Read the model definition and answer for the solid it produces. Units are mm, in the model's axes. Face numbers are marked on the shaded views. A direction names the side the tool comes from. Give positions to 0.01 mm unless a question says otherwise; leave off trailing zeros. Write each loop counter-clockwise with the first axis right and the second up, starting at its lowest first coordinate (ties: lowest second). Pieces come first, ordered by that corner, then holes. Notation, with made-up numbers: (63.5, 75) -> (101.5, 75) arc R23 cw to (101.5, 83) -> close; hole circle Ø5 at (67, -27.75). An arc over 180 degrees is marked (long way). Use a Markdown table: item, result.
Autodesk Inventor part; units mm, degrees
ref_plane "YZ Plane" through (0, 0, 0) normal (1, 0, 0) x (0, 1, 0)
ref_plane "XY Plane" through (0, 0, 0) normal (0, 0, 1) x (1, 0, 0)
sketch "Sketch1" plane through (0, 0, 0) normal (0, 0, 1) x (1, 0, 0)
  line L0 (0, 0) -> (1000, 0)
  line L1 (1000, 0) -> (1000, 1250)
  line L2 (1000, 1250) -> (0, 1250)
  line L3 (0, 1250) -> (0, 0)
  dimension "d0" = 1000
  dimension "d1" = 1250
extrude "Extrusion1" add sketch "Sketch1" along normal blind 100
sketch "Sketch2" plane through (0, 0, 0) normal (0, 0, -1) x (-1, 0, 0)
  line L0 (-1000, 1250) -> (0, 1250)
  circle A0 centre (-500, 1250) radius 500
  point P0 (0, 0)
  dimension "d4" = 1000
extrude "Extrusion2" add sketch "Sketch2" against normal blind 100 contours A0 L0 picked at (-386.6625, 1415.594)
sketch "Sketch3" plane through (0, 0, 0) normal (0, -1, 0) x (1, 0, 0)
  line L0 (0, 100) -> (1000, 100)
  circle A0 centre (350, 100) radius 50
  circle A1 centre (650, 100) radius 50
  line L1 (0, 0) -> (0, 100)
  line L2 (1000, 0) -> (1000, 100)
  point P0 (1000, 50)
  dimension "d7" = 100
  dimension "d8" = 100
  dimension "d9" = 350
  dimension "d10" = 350
extrude "Extrusion3" add sketch "Sketch3" against normal blind 1250
sketch "Sketch4" plane through (1000, 0, 100) normal (1, 0, 0) x (0, 0, -1)
  line L0 (0, 1250) -> (0, 0)
  circle A0 centre (0, 450) radius 50
  circle A1 centre (0, 850) radius 50
  line L1 (100, 0) -> (0, 0)
  line L2 (100, 1250) -> (0, 1250)
  dimension "d13" = 100
  dimension "d14" = 100
  dimension "d15" = 450
  dimension "d16" = 400
  dimension "d17" = 400
extrude "Extrusion4" add sketch "Sketch4" against normal blind 1000
sketch "Sketch5" plane through (0, 0, 100) normal (0, 0, 1) x (1, 0, 0)
  line L0 (700, 1250) -> (600, 1250)
  line L1 (400, 1250) -> (300, 1250)
  arc A0 (600, 1250) -> (400, 1250) centre (500, 1250) ccw
  arc A1 (700, 1250) -> (300.0458, 1245.6914) centre (500.0458, 1245.7187) ccw
  point P0 (0, 0)
  point P1 (300.0917, 1250)
  dimension "d20" = 100
  dimension "d21" = 200
extrude "Extrusion5" add sketch "Sketch5" along normal blind 50
sketch "Sketch6" plane through (1000, 0, 100) normal (1, 0, 0) x (0, 0, -1)
  line L0 (0, 900) -> (0, 1250)
  circle A0 centre (0, 1200) radius 50
  line L1 (100, 1250) -> (0, 1250)
  point P0 (100, 0)
  dimension "d24" = 100
  dimension "d25" = 50
extrude "Extrusion6" add sketch "Sketch6" against normal up to surface
sketch "Sketch7" plane through (0, 0, 0) normal (-1, 0, 0) x (0, 0, 1)
  line L0 (100, 900) -> (100, 1250)
  circle A0 centre (100, 1200) radius 50
  line L1 (0, 1250) -> (100, 1250)
  point P0 (0, 0)
  dimension "d28" = 100
  dimension "d29" = 50
extrude "Extrusion7" add sketch "Sketch7" against normal up to surface
ref_plane "Work Plane1" through (0, 1750, 0) normal (0, 1, 0) x (-1, 0, 0)
sketch "Sketch8" plane through (0, 1750, 0) normal (0, 1, 0) x (-1, 0, 0)
  line L0 (-400, 100) -> (-600, 100)
  circle A0 centre (-500, 100) radius 50
  point P0 (0, 0)
  dimension "d33" = 100
extrude "Extrusion8" add sketch "Sketch8" against normal up to surface
sketch "Sketch9" plane through (0, 0, 100) normal (0, 0, 1) x (1, 0, 0)
  line L0 (1000, 1150) -> (700, 1150)
  line L1 (900, 1150) -> (900, 902.0075)
  line L2 (1000, 900) -> (1000, 1150)
  line L3 (1000, 800) -> (700, 800)
  line L4 (900, 800) -> (900, 0)
  line L5 (0, 0) -> (1000, 0)
  line L6 (100, 0) -> (100, 1250)
  line L7 (0, 1250) -> (300, 1250)
  line L8 (0, 800) -> (0, 500)
  arc A0 (1000, 1250) -> (0, 1250) centre (500, 1250) ccw
  line L9 (0, 1250) -> (0, 0)
  line L10 (0, 1250) -> (0, 0)
  line L11 (700, 1250) -> (1000, 1250)
  line L12 (1000, 1250) -> (1000, 0)
  arc A1 (900, 1250) -> (100, 1250) centre (500, 1250) ccw
  point P0 (900, 1026.0038)
  point P1 (100, 625)
  dimension "d36" = 100
  dimension "d37" = 100
extrude "Extrusion9" add sketch "Sketch9" along normal blind 50 contours L11 A1 L7 A0
sketch "Sketch10" plane through (0, 0, 100) normal (0, 0, 1) x (1, 0, 0)
  arc A0 (900, 1250) -> (550, 1646.8627) centre (500, 1250) ccw
  line L0 (900, 1250) -> (900, 0)
  line L1 (1000, 0) -> (1000, 1250)
  line L2 (1000, 1250) -> (1000, 0)
  line L3 (1000, 1150) -> (700, 1150)
  line L4 (900, 1150) -> (1000, 1150)
  line L5 (0, 0) -> (1000, 0)
  line L6 (900, 0) -> (1000, 0)
extrude "Extrusion10" add sketch "Sketch10" along normal blind 50
sketch "Sketch11" plane through (0, 0, 100) normal (0, 0, 1) x (1, 0, 0)
  line L0 (100, 1250) -> (100, 0)
  line L1 (0, 0) -> (300, 0)
  line L2 (0, 0) -> (0, 1250)
  line L3 (0, 400) -> (0, 0)
  line L4 (0, 1250) -> (100, 1250)
  line L5 (0, 0) -> (100, 0)
extrude "Extrusion11" add sketch "Sketch11" along normal blind 50
sketch "Sketch12" plane through (0, 0, 100) normal (0, 0, 1) x (1, 0, 0)
  line L0 (700, 1250) -> (900, 1250)
  line L1 (900, 1250) -> (900, 1150)
  line L2 (900, 1150) -> (1000, 1150)
  line L3 (900, 1250) -> (1000, 1250)
  line L4 (1000, 1150) -> (1000, 1250)
  line L5 (1000, 1250) -> (900, 1250)
  point P0 (0, 0)
extrude "Extrusion12" add sketch "Sketch12" along normal blind 50
sketch "Sketch13" plane through (0, 0, 100) normal (0, 0, 1) x (1, 0, 0)
  line L0 (0, 1250) -> (0, 0)
  line L1 (0, 100) -> (1042, 100)
  line L2 (400, 0) -> (600, 0)
  line L3 (0, 0) -> (100, 0)
  line L4 (0, 100) -> (0, 0)
  line L5 (900, 0) -> (1000, 0)
  line L6 (0, 0) -> (1000, 0)
  line L7 (1000, 0) -> (1000, 100)
  line L8 (1000, 0) -> (1000, 1250)
  point P0 (500, 0)
  point P1 (521, 100)
  dimension "d46" = 100
extrude "Extrusion13" add sketch "Sketch13" along normal blind 50
sketch "Sketch14" plane through (0, 0, 0) normal (0, 0, -1) x (-1, 0, 0)
  arc A0 (-500, 1750) -> (-1000, 1250) centre (-500, 1250) ccw
  line L0 (-1000, 0) -> (-1000, 1250)
  line L1 (-1000, 1250) -> (-1000, 0)
  line L2 (0, 0) -> (-1000, 0)
  line L3 (-1000, 0) -> (0, 0)
  arc A1 (0, 1250) -> (-500, 1750) centre (-500, 1250) ccw
  line L4 (0, 0) -> (0, 1250)
  line L5 (0, 1250) -> (-1000, 1250)
  circle A2 centre (-500, 1250) radius 500
extrude "Extrusion14" add sketch "Sketch14" along normal blind 150
properties part number "WindowofShip11"
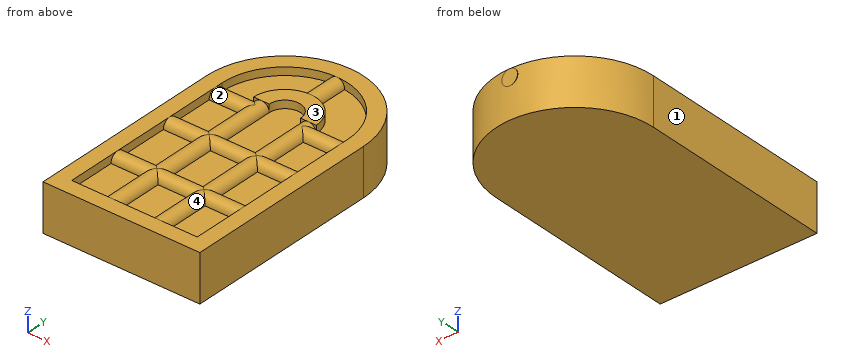
Item 1: For a pull along Y with two mould halves and no side action, classify the marked faces 3 and 4 as +Y half, -Y half, draft (parallel to the pull), parting line (faces both ways), or undercut.
Return value:
| item | result |
|---|---|
| face 3 | draft |
| face 4 | undercut |
Item 2: A tool of negligible diameter and unlimited length cuts with its end or side. For the marked faces 1 and 2, from which of +Z, -Z, +X, -X, +Y, -Y can it reach the whole face along a straight path? Write none if from no direction.
Return value:
| item | result |
|---|---|
| face 1 | +Z, -Z, -X, +Y, -Y |
| face 2 | +Z |
Item 3: A cutting plane is placed at B-B (z = -52). Give the vertices of the cut face in (x, y).
Return value:
| item | result |
|---|---|
| outline | (0, 0) -> (1000, 0) -> (1000, 1250) arc R500 ccw to (0, 1250) -> close |
Item 4: A cutting plane is placed at D-D (x = 258.5). Give the vertices of the cut face in (y, z), then the cut area to 3 significant figures.
Return value:
| item | result |
|---|---|
| outline | (0, -150) -> (1687.81, -150) -> (1687.81, 150) -> (1568.87, 150) -> (1568.87, 100) -> (1250, 100) arc R50 ccw to (1150, 100) -> (900, 100) arc R50 ccw to (800, 100) -> (500, 100) arc R50 ccw to (400, 100) -> (100, 100) -> (100, 150) -> (0, 150) -> close |
| area | 445,000 mm^2 |
Item 5: A cutting plane is placed at C-C (x = 768.5). Give the vertices of the cut face in (y, z), then the cut area to 3 significant figures.
Return value:
| item | result |
|---|---|
| outline | (0, -150) -> (1671.79, -150) -> (1671.79, 150) -> (1546.49, 150) -> (1546.49, 100) -> (1250, 100) arc R50 ccw to (1150, 100) -> (900, 100) arc R50 ccw to (800, 100) -> (500, 100) arc R50 ccw to (400, 100) -> (100, 100) -> (100, 150) -> (0, 150) -> close |
| area | 441,000 mm^2 |
Item 6: Each of these flat-tipped pins is pushed along its axis until it touches: P1, Ø15, axis at x = 431.5, z = 119, coming from the +Y side; P2, Ø4, axis at x = 733, z = -85.5, coming from the +Y side; P3, Ø6, axis at x = 629.5, y = 520.5, coming from the +Z side. Where does it stop, or does it pass through?
Return value:
| item | result |
|---|---|
| P1 | y = 1746.27 |
| P2 | y = 1693.44 |
| P3 | z = 146.84 |
Item 7: A cutting plane is placed at A-A (x = 425). Give the vertices of the cut face in (y, z).
Return value:
| item | result |
|---|---|
| outline | (0, -150) -> (1744.34, -150) -> (1744.34, 150) -> (1642.91, 150) -> (1642.91, 100) -> (1431.11, 100) -> (1431.11, 150) -> (1316.14, 150) -> (1316.14, 100) -> (900, 100) arc R50 ccw to (800, 100) -> (500, 100) arc R50 ccw to (400, 100) -> (100, 100) -> (100, 150) -> (0, 150) -> close |
Item 8: Straight lines are drawn through the part: line 1 along X through (y, z) = (1304, 133); line 2 along Z through (x, y) = (402, 1093.5); line 3 along Y through (x, z) = (564, 112). For each, find the intervals that lie inside material, in ascending order. Write a range as [from, to].
Return value:
| item | result |
|---|---|
| line 1 | [2.92, 103.66], [308.73, 415.83], [584.17, 691.37], [896.34, 997.08] |
| line 2 | [-150, 100] |
| line 3 | [0, 100], [401.46, 498.54], [801.46, 898.54], [1326.84, 1435.22], [1644.85, 1745.89] |
